```python
from build123d import *

# Parameters (mm, degrees)
SKETCH1_W           = 55
SKETCH1_H           = 55
SKETCH1_R           = 1.75
BOSS_EXTRUDE1_DEPTH = 3.5
SKETCH2_R           = 15
CUT_EXTRUDE1_DEPTH  = 40.048047326
SKETCH3_R           = 1.5
CUT_EXTRUDE2_DEPTH  = 40.048047326
CHAMFER1_SIZE       = 5


with BuildPart() as part:
    # Sketch1 → Boss-Extrude1 (new body)
    with BuildSketch(Plane.XY):
        Rectangle(SKETCH1_W, SKETCH1_H)
        with Locations((19.445436483, 19.445436483)):
            Circle(SKETCH1_R, mode=Mode.SUBTRACT)
        with Locations((-19.445436483, 19.445436483)):
            Circle(SKETCH1_R, mode=Mode.SUBTRACT)
        with Locations((-19.445436483, -19.445436483)):
            Circle(SKETCH1_R, mode=Mode.SUBTRACT)
        with Locations((19.445436483, -19.445436483)):
            Circle(SKETCH1_R, mode=Mode.SUBTRACT)
    extrude(amount=BOSS_EXTRUDE1_DEPTH)

    # Sketch2 → Cut-Extrude1 (cut, through all)
    with BuildSketch(Plane(origin=(0, 0, 0), x_dir=(-1, 0, 0), z_dir=(0, 0, -1))):
        Circle(SKETCH2_R)
    extrude(amount=-CUT_EXTRUDE1_DEPTH, mode=Mode.SUBTRACT)

    # Sketch3 → Cut-Extrude2 (cut, through all)
    with BuildSketch(Plane(origin=(0, 0, 0), x_dir=(-1, 0, 0), z_dir=(0, 0, -1))):
        with Locations((0, 21.920310217)):
            Circle(SKETCH3_R)
        with Locations((21.920310217, 0)):
            Circle(SKETCH3_R)
        with Locations((0, -21.920310217)):
            Circle(SKETCH3_R)
        with Locations((-21.920310217, 0)):
            Circle(SKETCH3_R)
    extrude(amount=-CUT_EXTRUDE2_DEPTH, mode=Mode.SUBTRACT)

    # Chamfer1
    chamfer1_edges = [part.edges().sort_by_distance(p)[0] for p in [
        (27.5, -27.5, 1.75),
        (-27.5, -27.5, 1.75),
        (-27.5, 27.5, 1.75),
        (27.5, 27.5, 1.75),
    ]]
    chamfer(chamfer1_edges, length=CHAMFER1_SIZE)


solid = part.part
```
Source: CAD feature listing. Evaluate the final solid. Frame: model axes, mm. Round coordinates to 2 decimals unless told otherwise and drop trailing zeros. Loops run counter-clockwise (first coordinate to the right, second up) from the corner with the lowest first, then second, coordinate; pieces in that order, holes last. Notation, with made-up numbers: M -33,21.25 L 5,21.25 A34 ccw 5,59.25 Z; hole C 74,67.25 d7. An arc over 180 degrees is marked long. Use a Markdown table: item, result. Add a question column.
1. Cut plane C-C, the plane y = 9. Output: boundary loops of the cut face in (x, z), and give its area (4 significant figures).
2. Cut plane D-D, the plane x = -8.5. Output: boundary loops of the cut face in (y, z), and give its area (3 significant figures).
3. Pull-direction query (X, two-part tool) for faces 1 (the flat face through (12, -12, 3.5)), 2 (the cylindrical face through (-20.42, 0.07, 1.73)), 3 (the flat face through (25, -25, 2)), 4 (the flat face through (-27.5, 0, 2)); classes: +X half, -X half, draft (parallel to the pull), parting line (faces both ways), or undercut.
4. Ray query, line 1 along Y through (x, z) = (0, 0.95); line 2 along X through (y, z) = (-0.5, 2.9); line 3 along X through (y, z) = (-19, 0.75). Return the intervals inside material, ascending. Write a range as [from, to].
5. Cut plane A-A, the plane y = 0. Output: boundary loops of the cut face in (x, z).
6. Contact query for a flat-ended pin moving along its axis: pin 1 (2.5 mm diameter, centred on x = -21.92, y = 0, fed in from -Z). Output: stop coordinate, or through.
Solution:
| question | item | result |
|---|---|---|
| 1 | outline | M -27.5,0 L -12,0 L -12,3.5 L -27.5,3.5 Z; M 12,0 L 27.5,0 L 27.5,3.5 L 12,3.5 Z |
| 1 | area | 108.5 mm2 |
| 2 | outline | M -27.5,0 L -12.36,0 L -12.36,3.5 L -27.5,3.5 Z; M 12.36,0 L 27.5,0 L 27.5,3.5 L 12.36,3.5 Z |
| 2 | area | 106 mm2 |
| 3 | face 1 | draft |
| 3 | face 2 | undercut |
| 3 | face 3 | +X half |
| 3 | face 4 | -X half |
| 4 | line 1 | y = [-27.5, -23.42], [-20.42, -15], [15, 20.42], [23.42, 27.5] |
| 4 | line 2 | x = [-27.5, -23.33], [-20.51, -14.99], [14.99, 20.51], [23.33, 27.5] |
| 4 | line 3 | x = [-27.5, -21.14], [-17.75, 17.75], [21.14, 27.5] |
| 5 | outline | M -27.5,0 L -23.42,0 L -23.42,3.5 L -27.5,3.5 Z; M -20.42,0 L -15,0 L -15,3.5 L -20.42,3.5 Z; M 15,0 L 20.42,0 L 20.42,3.5 L 15,3.5 Z; M 23.42,0 L 27.5,0 L 27.5,3.5 L 23.42,3.5 Z |
| 6 | pin 1 | passes through |
